The listing builds one solid part. Answer for the finished solid, in the listing's coordinates (mm). Coordinates: 2 decimals unless noted, no trailing zeros. Order: outer loops, then holes, each group sorted by start corner. A loop starts at its lowest first (then second) coordinate and runs counter-clockwise, first axis right, second up. Notation, with made-up numbers: (33, -32.75) - (64, -32.75) arc R25 ccw to (64, 5.25) - close; hole circle Ø2 at (24.25, -27). An arc over 180 degrees is marked (long way). Use one line per item in the form item = value. Start each with the question number.
Item 1: The mould has two halves that part along Y. Classify faces 1 (the flat face through (199, 203, 170)), 2 (the cylindrical face through (201.038, 198.004, 172.465)), 3 (the cylindrical face through (306.99, 202.15, 171.52)): released by +Y, released by -Y, zero draft, split by the parting line, or undercut.
Item 2: Consider line 1 along Y through (x, z) = (200, 171.95); line 2 along Y through (x, z) = (200, 171.4); line 3 along Y through (x, z) = (271, 171.65). Determine where each line is inside the solid, lowest interval first. Write a range as [from, to].
Item 3: This flat-tipped pin is pushed along its axis until it touches: pin 1 Ø1.5 at (y, z) = (203, 171.5) entering from -X. Where does it stop, or does it pass through?
Item 4: Section C-C, the plane x = 268.5 is taken. Write down the section's boundary in (y, z).
Item 5: Section A-A, the plane x = 200 is taken. Write down the section's boundary in (y, z), and give its area (3 significant figures).
from build123d import *

# Parameters (mm, degrees)
SKETCH28_W           = 220
SKETCH28_H           = 10
SKETCH28_R           = 2.25
BOSS_EXTRUDE11_DEPTH = 5
VARFILLET1_R         = 10
VARFILLET2_R         = 10
VARFILLET3_R         = 2
VARFILLET4_R         = 2


with BuildPart() as part:
    # Sketch28 → Boss-Extrude11 (new body)
    with BuildSketch(Plane.XY.offset(170)):
        with Locations((200, 200)):
            Rectangle(SKETCH28_W, SKETCH28_H)
        with Locations((200, 200)):
            Circle(SKETCH28_R, mode=Mode.SUBTRACT)
    extrude(amount=BOSS_EXTRUDE11_DEPTH)

    # VarFillet1
    varfillet1_edges = [part.edges().sort_by_distance(p)[0] for p in [
        (310, 205, 172.5),
    ]]
    fillet(varfillet1_edges, radius=VARFILLET1_R - 0.0001)  # a hair under: the kernel refuses the full size

    # VarFillet2
    varfillet2_edges = [part.edges().sort_by_distance(p)[0] for p in [
        (90, 195, 172.5),
    ]]
    fillet(varfillet2_edges, radius=VARFILLET2_R - 0.0001)  # a hair under: the kernel refuses the full size

    # VarFillet3
    varfillet3_edges = [part.edges().sort_by_distance(p)[0] for p in [
        (307.071097101, 202.071097101, 175),
    ]]
    fillet(varfillet3_edges, radius=VARFILLET3_R)

    # VarFillet4
    varfillet4_edges = [part.edges().sort_by_distance(p)[0] for p in [
        (92.928902899, 197.928902899, 170),
    ]]
    fillet(varfillet4_edges, radius=VARFILLET4_R)


solid = part.part
Response:
q1.face_1 = zero draft
q1.face_2 = undercut
q1.face_3 = released by +Y
q2.line_1 = [195, 197.75], [202.25, 205]
q2.line_2 = [195.09, 197.75], [202.25, 205]
q2.line_3 = [195.03, 205]
q3.pin_1 = 90.1
q4.outline = (195, 172) arc R2 ccw to (197, 170) - (205, 170) - (205, 173) arc R2 ccw to (203, 175) - (195, 175) - close
q5.outline = (195, 172) arc R2 ccw to (197, 170) - (197.75, 170) - (197.75, 175) - (195, 175) - close; (202.25, 170) - (205, 170) - (205, 173) arc R2 ccw to (203, 175) - (202.25, 175) - close
q5.area = 25.8 mm2
